```python
from build123d import *

# Parameters (mm, degrees)
F0_W     = 25.4
F0_H     = 25.4
F1_DEPTH = 50.8
F3_DEPTH = 12.7
F4_SIZE  = 1


with BuildPart() as f1:
    # F0 (on Front) → F1 (new body, symmetric)
    with BuildSketch(Plane.XZ):
        Rectangle(F0_W, F0_H)
    extrude(amount=F1_DEPTH, both=True)

    # F2 (on face) → F3 (cut)
    with BuildSketch(Plane.XY.offset(12.7)):
        with BuildLine():
            Line((-6.35, -6.35), (-6.35, -50.8))
            Line((-6.35, -50.8), (6.35, -50.8))
            Line((6.35, -50.8), (6.35, -6.35))
            ThreePointArc((6.35, -6.35), (0, 0), (-6.35, -6.35))
        make_face()
    extrude(amount=-F3_DEPTH, mode=Mode.SUBTRACT)

    # F4
    f4_edges = [f1.edges().sort_by_distance(p)[0] for p in [
        (12.7, 0, 12.7),
        (12.7, -50.8, 0),
        (12.7, 0, -12.7),
        (12.7, 50.8, 0),
        (0, 50.8, -12.7),
        (0, 50.8, 12.7),
        (-12.7, 50.8, 0),
        (-12.7, 0, 12.7),
        (-9.525, -50.8, 12.7),
        (9.525, -50.8, 12.7),
        (-12.7, 0, -12.7),
        (-12.7, -50.8, 0),
        (0, -50.8, -12.7),
    ]]
    chamfer(f4_edges, length=F4_SIZE)


solid = f1.part
```
The model under review builds one solid part; all positions refer to its coordinate system, in mm. A direction names the side the tool comes from. Coordinates: 2 decimals unless noted, no trailing zeros. Write each loop counter-clockwise with the first axis right and the second up, starting at its lowest first coordinate (ties: lowest second). Pieces come first, ordered by that corner, then holes. Notation, with made-up numbers: (-35, -22.5) -> (-12, -22.5) arc R21 cw to (-12, -17.5) -> close; hole circle Ø7 at (-38.75, 16.25). An arc over 180 degrees is marked (long way). One line per item, written item: value. Start each with the question number.
Q1. For faces 1 (the face through (0, -25, 0)), 2 (the face through (0, -1, -12.7)), list the 3-axis set-ups (+Z, -Z, +X, -X, +Y, -Y) from which the entire face can be reached by the end or side of a thin tool; tool diameter is ignored.
Q2. Add section C-C, the plane y = -2. Give the boundary of the cut face in (x, z).
Q3. To check wall thickness, follow probe 1 along X at (y, z) = (-9, 7); probe 2 along Z at (x, y) = (-5, -12.5). State the ranges of each line that lie inside material, in increasing order.
Q4. The part is to be moulded in two halves that separate along X. For faces 3 (the face through (12.7, -1, 0)), 4 (the face through (0, 50.8, 0)), 5 (the face through (6.35, -29, 6)), 6 (the face through (0, 0, 6)), say which applies: +X half, -X half, draft (parallel to the pull), parting line (faces both ways), or undercut.
Q5. Clearance check with a flat-ended pin moving along its axis: P1, Ø1, axis at x = 5.5, y = -28, coming from the +Z side. State where the tip first meets the part, or that it passes through.
Q6. Add section A-A, the plane z = 4. Give the boundary of the cut face in (x, y).
Q7. Add section B-B, the plane x = 0. Give the boundary of the cut face in (y, z), then the cut area to 3 significant figures.
Response:
1. face 1: +Z, -Y
1. face 2: -Z, +X, -X, +Y, -Y
2. outline: (-12.7, -11.7) -> (-11.7, -12.7) -> (11.7, -12.7) -> (12.7, -11.7) -> (12.7, 11.7) -> (11.7, 12.7) -> (4.63, 12.7) -> (4.63, 0) -> (-4.63, 0) -> (-4.63, 12.7) -> (-11.7, 12.7) -> (-12.7, 11.7) -> close
3. probe 1: -12.7 to -6.35, 6.35 to 12.7
3. probe 2: -12.7 to 0
4. face 3: +X half
4. face 4: draft
4. face 5: undercut
4. face 6: undercut
5. P1: z = 0
6. outline: (-12.7, -49.8) -> (-11.7, -50.8) -> (-6.35, -50.8) -> (-6.35, -6.35) arc R6.35 cw to (6.35, -6.35) -> (6.35, -50.8) -> (11.7, -50.8) -> (12.7, -49.8) -> (12.7, 49.8) -> (11.7, 50.8) -> (-11.7, 50.8) -> (-12.7, 49.8) -> close
7. outline: (-50.8, -11.7) -> (-49.8, -12.7) -> (49.8, -12.7) -> (50.8, -11.7) -> (50.8, 11.7) -> (49.8, 12.7) -> (0, 12.7) -> (0, 0) -> (-50.8, 0) -> close
7. area: 1,930 mm²
